Geometry: final body of the model. Coordinates: model frame, mm. A direction names the side the tool comes from. Give positions to 0.01 mm unless a question says otherwise; leave off trailing zeros. Write each loop counter-clockwise with the first axis right and the second up, starting at its lowest first coordinate (ties: lowest second). Pieces come first, ordered by that corner, then holes.
Q1. Reachability of faces 4 (the flat face through (1, 0, 4)), 5 (the flat face through (-1.016, 4, 0)) from +Z, -Z, +X, -X, +Y, -Y: full face, straight path, thin tool, end or side. Return the list, or none.
Q2. Line query: line 1 (Y direction, x = 0, z = 2); line 2 (X direction, y = 3.75, z = 3); line 3 (Y direction, x = -2.5, z = 3.75). Output: solid intervals per line, ascending.
Q3. Section A-A (x = 0). Return the cut outline in (y, z), plus the area to 3 significant figures.
Q4. Mould query, pull axis X, two halves, no side actions, for faces 1 (the cylindrical face through (-3.57, -11.07, 0.16)), 2 (the flat face through (1.016, 3, 0)), 3 (the flat face through (0, -21.844, 0)). Classes: +X half, -X half, draft (parallel to the pull), parting line (faces both ways), or undercut.
Q5. Pin query (flat end, axial travel): pin 1 Ø1.6 at (x, z) = (0, -1) entering from +Y; pin 2 Ø4 at (x, z) = (3, 2) entering from +Y; pin 3 Ø1 at (y, z) = (-12, 0.5) entering from -X. Return the tip coordinate at first contact, or that it passes through.
Q6. Section D-D (z = 3.25). Return the cut outline in (x, y), plus the area to 3 significant figures.
Q7. Section B-B (z = 1). Return the cut outline in (x, y), plus the area to 3 significant figures.
Q8. Section C-C (y = -11). Return the cut outline in (x, z).
from build123d import *

# Parameters (mm, degrees)
CUT_EXTRUDE1_DEPTH      = 24.028962914
CUT_EXTRUDE1_DEPTH_BACK = 24.028962914


with BuildPart() as part:
    # Sketch1 → Base-Revolve (revolve)
    with BuildSketch(Plane.XY):
        with BuildLine():
            Line((5.1562, 0), (3.571875, 0))
            Line((3.571875, 0), (3.571875, -21.844))
            Line((3.571875, -21.844), (0, -21.844))
            Line((0, -21.844), (0, 5.08))
            ThreePointArc((0, 5.08), (3.619143491, 3.596659144), (5.1562, 0))
        make_face()
    revolve(axis=Axis((0, 10.110523875, 0), (0, -1, 0)))

    # Sketch2 → Cut-Extrude1 (cut, two sides: drawn at the far end of the back side and taken through both)
    with BuildSketch(Plane.XY.offset(-CUT_EXTRUDE1_DEPTH_BACK)):
        with BuildLine():
            Line((-1.016, 4.978921954), (-1.016, 2.54))
            Line((-1.016, 2.54), (1.016, 2.54))
            Line((1.016, 2.54), (1.016, 4.978921954))
            ThreePointArc((1.016, 4.978921954), (0, 5.08), (-1.016, 4.978921954))
        make_face()
    extrude(amount=CUT_EXTRUDE1_DEPTH + CUT_EXTRUDE1_DEPTH_BACK, mode=Mode.SUBTRACT)


solid = part.part
Computed:
1. face 4: -Y
1. face 5: +Z, -Z, +Y
2. line 1: y = -21.84 to 2.54
2. line 2: x = -1.72 to -1.02, 1.02 to 1.72
2. line 3: y = 0 to 2.43
3. outline: (-21.84, -3.57) - (0, -3.57) - (0, -5.16) arc R5.16 ccw to (2.54, -4.44) - (2.54, 4.44) arc R5.16 ccw to (0, 5.16) - (0, 3.57) - (-21.84, 3.57) - close
3. area: 181 mm2
4. face 1: parting line
4. face 2: undercut
4. face 3: draft
5. pin 1: stops at y = 2.54
5. pin 2: stops at y = 4.82
5. pin 3: stops at x = -3.57
6. outline: (-4, 0) - (-1.48, 0) - (-1.48, -21.84) - (1.48, -21.84) - (1.48, 0) - (4, 0) arc R4 ccw to (1.02, 3.8) - (1.02, 2.54) - (-1.02, 2.54) - (-1.02, 3.8) arc R4 ccw to start
6. area: 86.6 mm2
7. outline: (-5.06, 0) - (-3.43, 0) - (-3.43, -21.84) - (3.43, -21.84) - (3.43, 0) - (5.06, 0) arc R5.06 ccw to (1.02, 4.88) - (1.02, 2.54) - (-1.02, 2.54) - (-1.02, 4.88) arc R5.06 ccw to start
7. area: 184 mm2
8. outline: circle Ø7.14 at (0, 0)
